Geometry check sheet. Reference: the model listing, model coordinates, mm. A direction names the side the tool comes from. Coordinates: 2 decimals unless noted, no trailing zeros. Loops run counter-clockwise (first coordinate to the right, second up) from the corner with the lowest first, then second, coordinate; pieces in that order, holes last.
from build123d import *

# Parameters (mm, degrees)
SKETCH_1_R          = 2.5
EXTRUDE_1_DEPTH     = 25
EXTRUDE_2_DEPTH     = 8
EXTRUDE_3_DEPTH     = 8
CHAMFER_1_SIZE      = 1
SKETCH_4_R          = 1.25
CUT_EXTRUDE_1_DEPTH = 8
CUT_EXTRUDE_START   = 8
SKETCH_5_R          = 1.25
CUT_EXTRUDE_2_DEPTH = 8


with BuildPart() as part:
    # 草图1 → 凸台-拉伸1 (new body)
    with BuildSketch(Plane(origin=(0, 0, 0), x_dir=(1, 0, 0), z_dir=(0, 1, 0))):
        with Locations(Location((0, 0, 0), (0, 0, 270))):
            Circle(SKETCH_1_R)
    extrude(amount=EXTRUDE_1_DEPTH)

    # 草图2 → 凸台-拉伸2 (add)
    with BuildSketch(Plane(origin=(0, 25, 0), x_dir=(1, 0, 0), z_dir=(0, 1, 0))):
        Polygon((3.202903935, -1.319623577), (2.744279509, 2.113984385), (-0.458624426, 3.433607962), (-3.202903935, 1.319623577), (-2.744279509, -2.113984385), (0.458624426, -3.433607962), align=None)
    extrude(amount=-EXTRUDE_2_DEPTH)

    # 草图3 → 凸台-拉伸3 (add)
    with BuildSketch(Plane.XZ):
        Polygon((3.202903935, 1.319623577), (0.458624426, 3.433607962), (-2.744279509, 2.113984385), (-3.202903935, -1.319623577), (-0.458624426, -3.433607962), (2.744279509, -2.113984385), align=None)
    extrude(amount=-EXTRUDE_3_DEPTH)

    # 倒角1
    # the kernel refuses this chamfer: 1 mm, written as the material it adds along each edge
    with BuildSketch(Plane(origin=(0, 17, 0), x_dir=(0, 0, 1), z_dir=(1, 0, 0))) as chamfer_1_piece_1_section:
        Polygon((2.5, CHAMFER_1_SIZE), (2.5 + CHAMFER_1_SIZE, 0), (2.5, 0), align=None)
    chamfer_1_piece_1 = revolve(axis=Axis((0, 17, 0), (0, -1, 0)), mode=Mode.PRIVATE)
    chamfer_1_piece_1 = split(chamfer_1_piece_1, bisect_by=Plane(origin=(2.585980682, 16.482096178, -3.299128656), z_dir=(-0.9911972405355005, 0, 0.13239346794615373)), keep=Keep.TOP, mode=Mode.PRIVATE)
    chamfer_1_piece_1 = split(chamfer_1_piece_1, bisect_by=Plane(origin=(3.258731824, 16.482096178, 1.276618014), z_dir=(-0.61025472680424, 0, -0.7922052564917015)), keep=Keep.TOP, mode=Mode.PRIVATE)
    chamfer_1_piece_1 = split(chamfer_1_piece_1, bisect_by=Plane(origin=(0.102470937, 16.482096178, -3.202431915), z_dir=(-0.3809425137312606, 0, 0.924598724437855)), keep=Keep.TOP, mode=Mode.PRIVATE)
    chamfer_1_piece_1 = split(chamfer_1_piece_1, bisect_by=Plane(origin=(-2.183184145, 16.482096178, 2.345160432), z_dir=(0.38094251373126053, 0, -0.924598724437855)), keep=Keep.TOP, mode=Mode.PRIVATE)
    chamfer_1_piece_1 = split(chamfer_1_piece_1, bisect_by=Plane(origin=(-0.402796537, 16.482096178, -3.476613525), z_dir=(0.6102547268042401, 0, 0.7922052564917015)), keep=Keep.TOP, mode=Mode.PRIVATE)
    chamfer_1_piece_1 = split(chamfer_1_piece_1, bisect_by=Plane(origin=(-3.361202761, 16.482096178, -2.504767848), z_dir=(0.9911972405355005, 0, -0.1323934679461537)), keep=Keep.TOP, mode=Mode.PRIVATE)
    add(chamfer_1_piece_1)
    with BuildSketch(Plane(origin=(0, 8, 0), x_dir=(0, 0, 1), z_dir=(1, 0, 0))) as chamfer_1_piece_2_section:
        Polygon((2.5 + CHAMFER_1_SIZE, 0), (2.5, -CHAMFER_1_SIZE), (2.5, 0), align=None)
    chamfer_1_piece_2 = revolve(axis=Axis((0, 8, 0), (0, -1, 0)), mode=Mode.PRIVATE)
    chamfer_1_piece_2 = split(chamfer_1_piece_2, bisect_by=Plane(origin=(3.258731824, 8.517903822, 1.276618014), z_dir=(-0.61025472680424, 0, -0.7922052564917015)), keep=Keep.TOP, mode=Mode.PRIVATE)
    chamfer_1_piece_2 = split(chamfer_1_piece_2, bisect_by=Plane(origin=(2.585980682, 8.517903822, -3.299128656), z_dir=(-0.9911972405355005, 0, 0.13239346794615373)), keep=Keep.TOP, mode=Mode.PRIVATE)
    chamfer_1_piece_2 = split(chamfer_1_piece_2, bisect_by=Plane(origin=(-2.183184145, 8.517903822, 2.345160432), z_dir=(0.38094251373126053, 0, -0.924598724437855)), keep=Keep.TOP, mode=Mode.PRIVATE)
    chamfer_1_piece_2 = split(chamfer_1_piece_2, bisect_by=Plane(origin=(0.102470937, 8.517903822, -3.202431915), z_dir=(-0.3809425137312606, 0, 0.924598724437855)), keep=Keep.TOP, mode=Mode.PRIVATE)
    chamfer_1_piece_2 = split(chamfer_1_piece_2, bisect_by=Plane(origin=(-3.361202761, 8.517903822, -2.504767848), z_dir=(0.9911972405355005, 0, -0.1323934679461537)), keep=Keep.TOP, mode=Mode.PRIVATE)
    chamfer_1_piece_2 = split(chamfer_1_piece_2, bisect_by=Plane(origin=(-0.402796537, 8.517903822, -3.476613525), z_dir=(0.6102547268042401, 0, 0.7922052564917015)), keep=Keep.TOP, mode=Mode.PRIVATE)
    add(chamfer_1_piece_2)

    # 草图4 → 切除-拉伸1 (cut)
    with BuildSketch(Plane(origin=(0, 0, 0), x_dir=(-1, 0, 0), z_dir=(0, 1, 0))):
        with Locations(Location((0, 0, 0), (0, 0, 90))):
            Circle(SKETCH_4_R)
    extrude(amount=CUT_EXTRUDE_1_DEPTH, mode=Mode.SUBTRACT)

    # 草图5 → 切除-拉伸2 (cut)
    with BuildSketch(Plane(origin=(0, 25, 0), x_dir=(-1, 0, 0), z_dir=(0, -1, 0)).offset(CUT_EXTRUDE_START)):
        with Locations(Location((0, 0, 0), (0, 0, 270))):
            Circle(SKETCH_5_R)
    extrude(amount=-CUT_EXTRUDE_2_DEPTH, mode=Mode.SUBTRACT)


solid = part.part
1) Mould release check, pull along X, two halves, no side actions. Record for faces 4 (the flat face through (-1.5, 0, 0)), 5 (the cylindrical face through (-2.44, 12.45, -0.54)), 6 (the cylindrical face through (1.22, 20.94, -0.27)): +X half, -X half, draft (parallel to the pull), parting line (faces both ways), or undercut.
Data:
face 4: draft
face 5: parting line
face 6: undercut
2) Section check A-A on y = 23.5. Record the cut outline in (x, z), and give its area (3 significant figures).
Data:
outline: (-3.2, -1.32) - (-0.46, -3.43) - (2.74, -2.11) - (3.2, 1.32) - (0.46, 3.43) - (-2.74, 2.11) - close; hole circle Ø2.5 at (0, 0)
area: 26.3 mm2
3) Depth check by flat-ended pin: pin 1 (2 mm diameter, centred on y = 5, z = -2.5, fed in from -X); pin 2 (1 mm diameter, centred on y = 11.5, z = -2, fed in from -X); pin 3 (3 mm diameter, centred on y = 8.5, z = 2.5, fed in from -X). Enter the tip coordinate at first touch or a pass-through.
Data:
pin 1: stops at x = -2.97
pin 2: stops at x = -2
pin 3: stops at x = -2.89
4) Access from +Z, -Z, +X, -X, +Y, -Y to the whole of each face (thin tool, end or side, straight path). Record for faces 1 (the flat face through (1, 25, -1)), 2 (the flat face through (0, 17, 0)), 3 (the cylindrical face through (-1.22, 3.94, -0.27)).
Data:
face 1: +Z, -Z, +X, -X, +Y
face 2: +Y
face 3: -Y
5) Material ranges on probe 1 along Y at (x, z) = (2.25, -1.25); probe 2 along X at (y, z) = (6.25, 0); probe 3 along Z at (x, y) = (0.5, 4.75), recorded low to high.
Data:
probe 1: y = 0 to 8.93, 16.07 to 25
probe 2: x = -3.03 to -1.25, 1.25 to 3.03
probe 3: z = -3.04 to -1.15, 1.15 to 3.4
6) Section check D-D on y = 13.25. Record the cut outline in (x, z).
Data:
outline: circle Ø5 at (0, 0)
7) Section check C-C on x = 0. Record the cut outline in (y, z).
Data:
outline: (0, -3.24) - (8.26, -3.24) - (9, -2.5) - (16, -2.5) - (16.74, -3.24) - (25, -3.24) - (25, -1.25) - (17, -1.25) - (17, 1.25) - (25, 1.25) - (25, 3.24) - (16.74, 3.24) - (16, 2.5) - (9, 2.5) - (8.26, 3.24) - (0, 3.24) - (0, 1.25) - (8, 1.25) - (8, -1.25) - (0, -1.25) - close
8) Section check B-B on z = 0. Record the cut outline in (x, y), and give its area (3 significant figures).
Data:
outline: (-3.03, 0) - (-1.25, 0) - (-1.25, 8) - (1.25, 8) - (1.25, 0) - (3.03, 0) - (3.03, 8.47) - (2.5, 9) - (2.5, 16) - (3.03, 16.53) - (3.03, 25) - (1.25, 25) - (1.25, 17) - (-1.25, 17) - (-1.25, 25) - (-3.03, 25) - (-3.03, 16.53) - (-2.5, 16) - (-2.5, 9) - (-3.03, 8.47) - close
area: 103 mm2
